The model under review builds one solid part; all positions refer to its coordinate system, in mm. Face numbers are marked on the shaded views. Give positions to 0.01 mm unless a question says otherwise; leave off trailing zeros. Loops run counter-clockwise (first coordinate to the right, second up) from the corner with the lowest first, then second, coordinate; pieces in that order, holes last. Notation, with made-up numbers: M 39.5,-34 L 81.5,-34 A10 cw 81.5,-29 Z; hole C -5.5,-30.5 d4. An arc over 180 degrees is marked long. Write item = value, one per line. Start each with the question number.
1. Wall thickness on line 1 along Z through (x, y) = (0, -19); line 2 along X through (y, z) = (3.75, 0); line 3 along Y through (x, z) = (-64.5, -47) (3 decimals): over which ranges is each line inside the solid? List them lowest first. Write a range as from..to.
2. We need section A-A on y = 2. Give the boundary of the cut face in (x, z), then the cut area to 3 significant figures.
3. We need section B-B on y = -11. Give the boundary of the cut face in (x, z), then the cut area to 3 significant figures.
4. For pin 1 (1 mm diameter, centred on x = -26.5, y = -7, fed in from -Z); pin 2 (2 mm diameter, centred on y = -24.5, z = -39.5, fed in from -X); pin 3 (1.9 mm diameter, centred on x = -39.64, z = -68.66, fed in from +Y), all flat-tipped, find the tip position at first contact; note any pin that passes through.
5. Draft analysis for pull direction Z (two halves, no side actions). For the marked faces 1 and 2, state which applies: pulls with the +Z half, pulls with the -Z half, needs draft (parallel to the pull), parting line crosses it, or undercut.
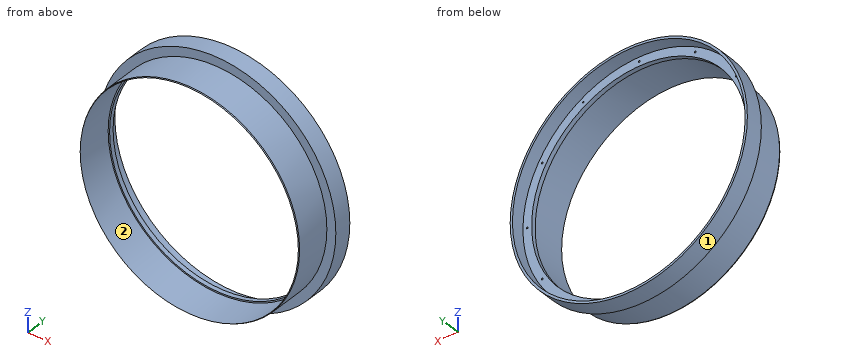
from build123d import *

# Parameters (mm, degrees)
SCREW_HOLES_COUNT = 12


with BuildPart() as part:
    # Cross Section → Main (revolve)
    with BuildSketch(Plane.XY):
        Polygon((-76.2, 0), (-76.2, -3.175), (-77.216, -3.175), (-77.216, -28.575), (-77.597, -27.915088642), (-77.597, -3.175), (-83.947, -3.175), (-83.947, 9.525), (-82.3595, 9.525), (-82.3595, 0), align=None)
    revolve(axis=Axis((0, 55, 0), (0, -1, 0)))

    # Sketch7 → #0-80 Tapped Hole1 (revolve, cut)
    with BuildSketch(Plane(origin=(-79.27975, 0, 0), x_dir=(0, 0, 1), z_dir=(1, 0, 0))):
        Polygon((0, 0), (0, 2.897890611), (0.59563, 2.54), (0.59563, 0), align=None)
    f_0_80_tapped_hole1 = revolve(axis=Axis((-79.27975, 6.35, 0), (0, -1, 0)), mode=Mode.SUBTRACT)

    # Screw Holes: #0-80 Tapped Hole1 ×12 about axis
    screw_holes_axis = Axis((0, 0, 0), (0, 1, 0))
    for i in range(1, SCREW_HOLES_COUNT):
        add(f_0_80_tapped_hole1.rotate(screw_holes_axis, i * 360 / SCREW_HOLES_COUNT), mode=Mode.SUBTRACT)


solid = part.part
Final values:
q1.line_1 = -77.6..-77.22, 77.22..77.6
q1.line_2 = -83.95..-82.36, 82.36..83.95
q1.line_3 = -3.175..0
q2.outline = C 0,0 d167.89; hole C 0,0 d164.72
q2.area = 829 mm²
q3.outline = C 0,0 d155.19; hole C 0,0 d154.43
q3.area = 185 mm²
q4.pin_1 = -73.11
q4.pin_2 = -67.37
q4.pin_3 = 0
q5.face_1 = parting line crosses it
q5.face_2 = undercut
